Input: part model. Units: mm. Frame: model coordinates. Face numbers are marked on the shaded views. Round coordinates to 2 decimals unless told otherwise and drop trailing zeros. Order: outer loops, then holes, each group sorted by start corner. A loop starts at its lowest first (then second) coordinate and runs counter-clockwise, first axis right, second up. Notation, with made-up numbers: (41, -6.5) -> (66, -6.5) arc R10 ccw to (66, 8.5) -> close; hole circle Ø5 at (-30, 58.5). An arc over 180 degrees is marked (long way). Use a Markdown table: item, result.
Autodesk Inventor part; units mm, degrees
ref_plane "YZ Plane" through (0, 0, 0) normal (1, 0, 0) x (0, 1, 0)
ref_plane "XZ Plane" through (0, 0, 0) normal (0, 1, 0) x (-1, 0, 0)
ref_plane "XY Plane" through (0, 0, 0) normal (0, 0, 1) x (1, 0, 0)
sketch "Sketch1" plane through (0, 0, 0) normal (0, 1, 0) x (-1, 0, 0)
  circle A0 centre (3.4811, 6.9947) radius 6.35
  line L0 (-9.2189, 19.6947) -> (16.1811, 19.6947)
  line L1 (16.1811, 19.6947) -> (16.1811, -18.4053)
  line L2 (16.1811, -18.4053) -> (-9.2189, -18.4053)
  line L3 (-9.2189, -18.4053) -> (-9.2189, 19.6947)
  point P0 (0, 0)
  dimension "d0" = 12.7
  dimension "d1" = 25.4
  dimension "d2" = 38.1
  dimension "d3" = 12.7
  dimension "d4" = 12.7
extrude "Extrusion1" add sketch "Sketch1" along normal blind 50.8 contours A0 | L0 L1 L2 L3
extrude "Extrusion2" cut sketch "Sketch1" along normal blind 44.45 contours A0
draft "FaceDraft1" angle 1 pull direction (0, -1, 0) faces at (9.2189, 16.9333, 6.9947) (-16.1811, 16.9333, -5.7053) (-7.7145, 33.8667, 19.6947) (-9.7489, 29.6333, 5.9761) fixed edges at (9.2189, 0, 0.6447) (-16.1811, 0, 0.6447) (-3.4811, 0, 19.6947) (2.8689, 0, 6.9947)
properties part number "Cylinder Cast Image"
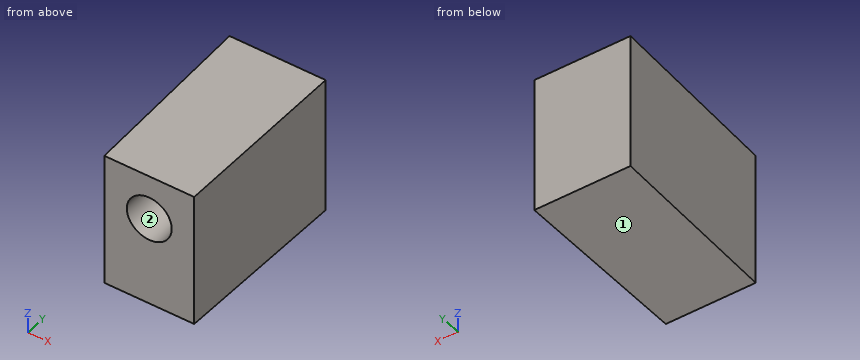
1) Draft query along X for the marked faces 1 and 2. Return one class per face: released by +X, released by -X, zero draft, split by the parting line, or undercut.
Answer key:
| item | result |
|---|---|
| face 1 | zero draft |
| face 2 | undercut |
2) Cut plane B-B on z = -2.5. Return loops of the section in (x, y), and give its area (3 significant figures).
Answer key:
| item | result |
|---|---|
| outline | (-17.07, 50.8) -> (-16.18, 0) -> (9.22, 0) -> (10.11, 50.8) -> close |
| area | 1,340 mm^2 |
3) Cut plane C-C on y = 39. Return loops of the section in (x, z).
Answer key:
| item | result |
|---|---|
| outline | (-16.86, -18.41) -> (9.9, -18.41) -> (9.9, 20.38) -> (-16.86, 20.38) -> close; hole circle Ø11.34 at (-3.48, 6.99) |
4) Cut plane A-A on y = 33. Return loops of the section in (x, z), and give its area (3 significant figures).
Answer key:
| item | result |
|---|---|
| outline | (-16.76, -18.41) -> (9.79, -18.41) -> (9.79, 20.27) -> (-16.76, 20.27) -> close; hole circle Ø11.55 at (-3.48, 6.99) |
| area | 922 mm^2 |
5) Contact query for flat-ended pins moving along their axis: P1, Ø5.5, axis at x = -5, z = 7.5, coming from the -Y side; P2, Ø8, axis at x = -3, y = 37.5, coming from the +Z side; P3, Ø3, axis at y = 24.5, z = 0.5, coming from the -X side. Output: stop coordinate, or through.
Answer key:
| item | result |
|---|---|
| P1 | stops at y = 44.45 |
| P2 | stops at z = 20.42 |
| P3 | stops at x = -16.63 |
6) Ray query, probe 1 along Y at (x, z) = (-6.5, 6); probe 2 along Z at (x, y) = (-6.25, 37); probe 3 along X at (y, z) = (19, 8.5). Return the intervals inside material, ascending.
Answer key:
| item | result |
|---|---|
| probe 1 | y = 44.45 to 50.8 |
| probe 2 | z = -18.41 to 2.01, 11.98 to 20.34 |
| probe 3 | x = -16.51 to -9.31, 2.35 to 9.55 |
